```python
from build123d import *

# Parameters (mm, degrees)
F0_W     = 130
F0_H     = 100
F1_DEPTH = 10
F3_D     = 9
F3_DEPTH = 9
F3_TIP   = 2.7038727856
F2_R     = 4
F4_DEPTH = 25
F5_DEPTH = 25
F6_DEPTH = 25
F7_DEPTH = 25
F8_D     = 7
F8_DEPTH = 5
F8_TIP   = 2.1030121666


with BuildPart() as f1:
    # F0 (on Front) → F1 (new body)
    with BuildSketch(Plane.XZ):
        with Locations((-9.0617658345, 20.0177619606)):
            Rectangle(F0_W, F0_H)
    extrude(amount=F1_DEPTH)

    # F3
    with Locations(Plane(origin=(0, 0, 0), x_dir=(-1, 0, 0), z_dir=(0, 1, 0))):
        with Locations((44.0617658345, 60.0177619606)):
            Hole(F3_D / 2, depth=F3_DEPTH)
            with Locations((0, 0, -(F3_DEPTH + F3_TIP / 2))):  # 118° drill point
                Cone(0, F3_D / 2, F3_TIP, mode=Mode.SUBTRACT)

    # F2 (on face) → F4 (cut)
    with BuildSketch(Plane(origin=(0, 0, 0), x_dir=(-1, 0, 0), z_dir=(0, 1, 0))):
        with Locations((-45.9382341655, -19.9822380394)):
            Circle(F2_R)
    extrude(amount=-F4_DEPTH, mode=Mode.SUBTRACT)

    # F2 (on face) → F5 (cut)
    with BuildSketch(Plane(origin=(0, 0, 0), x_dir=(-1, 0, 0), z_dir=(0, 1, 0))):
        with Locations((64.0617658345, -19.9822380394)):
            Circle(F2_R)
    extrude(amount=-F5_DEPTH, mode=Mode.SUBTRACT)

    # F2 (on face) → F6 (cut)
    with BuildSketch(Plane(origin=(0, 0, 0), x_dir=(-1, 0, 0), z_dir=(0, 1, 0))):
        with Locations((64.0617658345, 60.0177619606)):
            Circle(F2_R)
    extrude(amount=-F6_DEPTH, mode=Mode.SUBTRACT)

    # F2 (on face) → F7 (cut)
    with BuildSketch(Plane(origin=(0, 0, 0), x_dir=(-1, 0, 0), z_dir=(0, 1, 0))):
        with Locations((-45.9382341655, 60.0177619606)):
            Circle(F2_R)
    extrude(amount=-F7_DEPTH, mode=Mode.SUBTRACT)

    # F8
    with Locations(Plane(origin=(0, 0, 0), x_dir=(-1, 0, 0), z_dir=(0, 1, 0))):
        with Locations((9.0617658345, 0)):
            Hole(F8_D / 2, depth=F8_DEPTH)
            with Locations((0, 0, -(F8_DEPTH + F8_TIP / 2))):  # 118° drill point
                Cone(0, F8_D / 2, F8_TIP, mode=Mode.SUBTRACT)


solid = f1.part
```
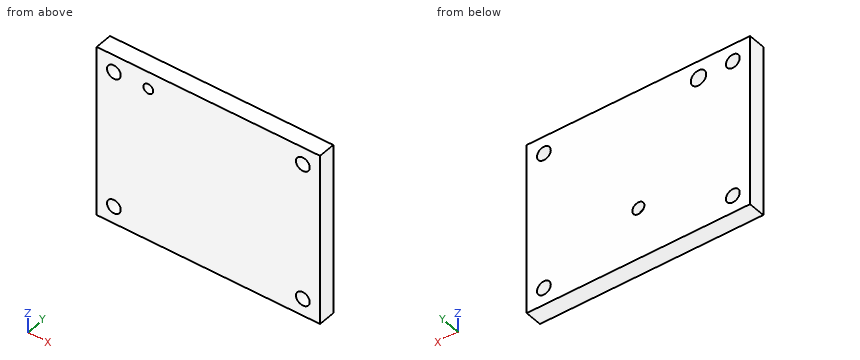
Design review of the part built by this model. Coordinates are the model's own, in mm. Give positions to 0.01 mm unless a question says otherwise; leave off trailing zeros. Write each loop counter-clockwise with the first axis right and the second up, starting at its lowest first coordinate (ties: lowest second). Pieces come first, ordered by that corner, then holes. Notation, with made-up numbers: (52.5, 81.5) - (75.5, 81.5) arc R8 ccw to (75.5, 87.5) - close; hole circle Ø4 at (-18, -19). An arc over 180 degrees is marked (long way). Return JSON: item names as keys, results as strings. Group by question number.
(1) To check wall thickness, follow probe 1 along Z at (x, y) = (-63, -9); probe 2 along X at (y, z) = (-8.75, -18.5); probe 3 along X at (y, z) = (-0.75, 3). State the ranges of each line that lie inside material, in increasing order.
(2) We need section B-B, the plane z = -22. Give the boundary of the cut face in (x, y), then the cut area to 3 significant figures.
(3) We need section A-A, the plane x = 45.5. Give the boundary of the cut face in (y, z), then the cut area to 3 significant figures.
(4) We need section C-C, the plane z = 57.5. Give the number of separate pieces and of enclosed holes in the cut face, then the cut area to 3 significant figures.
(5) Insertion check: pin 1 (13 mm diameter, centred on x = 45.94, z = 60.02, fed in from +Y); pin 2 (5.5 mm diameter, centred on x = -9.06, z = 0, fed in from +Y); pin 3 (8 mm diameter, centred on x = -44.06, z = 60.02, fed in from +Y). Each pin has a flat end and moves straight along its axis. Give the tip position at first contact, or say it passes through.
Reported:
{
 "1": {"probe 1": "z = -29.98 to -23.84, -16.13 to 56.16, 63.87 to 70.02", "probe 2": "x = -74.06 to -67.78, -60.35 to 42.22, 49.65 to 55.94", "probe 3": "x = -74.06 to -10.86, -7.26 to 55.94"},
 "2": {"outline": "(-74.06, -10) - (-67.52, -10) - (-67.52, 0) - (-74.06, 0) - close; (-60.61, -10) - (42.48, -10) - (42.48, 0) - (-60.61, 0) - close; (49.39, -10) - (55.94, -10) - (55.94, 0) - (49.39, 0) - close", "area": "1,160 mm2"},
 "3": {"outline": "(-10, -29.98) - (0, -29.98) - (0, -23.96) - (-10, -23.96) - close; (-10, -16.01) - (0, -16.01) - (0, 56.04) - (-10, 56.04) - close; (-10, 63.99) - (0, 63.99) - (0, 70.02) - (-10, 70.02) - close", "area": "841 mm2"},
 "4": {"separate pieces": "4", "enclosed holes": "0", "area": "1,100 mm2"},
 "5": {"pin 1": "stops at y = 0", "pin 2": "stops at y = -5.45", "pin 3": "stops at y = -9.3"}
}
